from build123d import *

# Parameters (mm, degrees)
SKETCH015_W  = 9.5
SKETCH015_H  = 4.5
PAD007_DEPTH = 10
SKETCH014_W  = 0.5
SKETCH014_H  = 0.5
PAD008_DEPTH = 0.4
SKETCH017_W  = 0.5
SKETCH017_H  = 4.9
PAD010_DEPTH = 0.5


with BuildPart() as part:
    # Sketch015 → Pad007 (new body)
    with BuildSketch(Plane.XY):
        Rectangle(SKETCH015_W, SKETCH015_H)
    extrude(amount=PAD007_DEPTH)

    # Sketch014 (on Face3 of Pad007) → Pad008 (join)
    with BuildSketch(Plane.XZ.offset(2.25)):
        with Locations((-4.5, 9.75)):
            Rectangle(SKETCH014_W, SKETCH014_H)
        with Locations((4.5, 9.75)):
            Rectangle(SKETCH014_W, SKETCH014_H)
    extrude(amount=PAD008_DEPTH)

    # Sketch017 (on Face4 of Pad008) → Pad010 (join)
    with BuildSketch(Plane(origin=(0, 0, 0), x_dir=(1, 0, 0), z_dir=(0, 0, -1))):
        with Locations((-4.5, 0.2)):
            Rectangle(SKETCH017_W, SKETCH017_H)
        with Locations((4.5, 0.2)):
            Rectangle(SKETCH017_W, SKETCH017_H)
    extrude(amount=PAD010_DEPTH)


solid = part.part
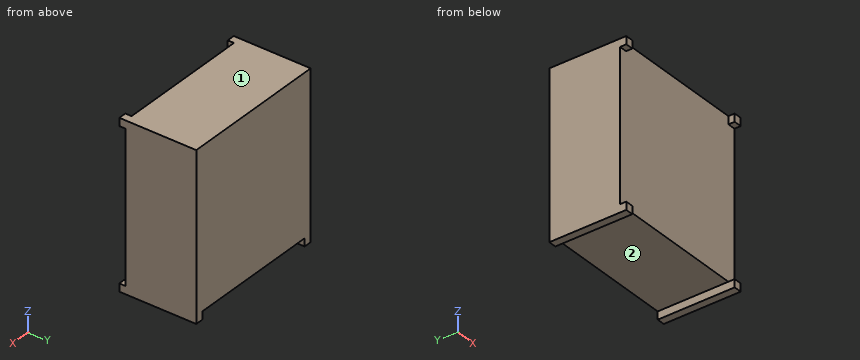
Could you check a few things on this model? Use its own coordinates, in mm. Face numbers are marked on the shaded views. A direction names the side the tool comes from. Round coordinates to 2 decimals unless told otherwise and drop trailing zeros. Loops run counter-clockwise (first coordinate to the right, second up) from the corner with the lowest first, then second, coordinate; pieces in that order, holes last. Notation, with made-up numbers: (54, 30.25) - (105, 30.25) arc R19 ccw to (105, 35.25) - close; hole circle Ø3 at (-17, 5.5). An arc over 180 degrees is marked (long way). Write item = value, one per line.
1) I need wall thicknesses on line 1 along Z through (x, y) = (-3.25, 2.05); line 2 along Y through (x, z) = (-0.25, 6.5). Which ranges of each line are inside material? Lowest first, please. Write a range as from..to.
Computed:
line_1 = 0..10
line_2 = -2.25..2.25
2) On a 3-axis mill with a long thin cutter (end or side, diameter ignored), from which of +Z, -Z, +X, -X, +Y, -Y can I reach the whole of each face in a straight line? I mean the marked faces 1 and 2. Say none if no direction works.
Computed:
face_1 = +Z, +X, -X, +Y, -Y
face_2 = -Z, +Y, -Y
3) Imagine slicing it at C-C (z = 5.25). Please give me the cut outline in (x, y), and give its area (4 significant figures).
Computed:
outline = (-4.75, -2.25) - (4.75, -2.25) - (4.75, 2.25) - (-4.75, 2.25) - close
area = 42.75 mm2
4) Imagine slicing it at A-A (y = -1.1). Please give me the cut outline in (x, z).
Computed:
outline = (-4.75, -0.5) - (-4.25, -0.5) - (-4.25, 0) - (4.25, 0) - (4.25, -0.5) - (4.75, -0.5) - (4.75, 10) - (-4.75, 10) - close
5) I'm going to push flat-ended pins straight in: P1, Ø2, axis at x = -0.5, y = 0, coming from the -Z side; P2, Ø1, axis at x = 3, z = 8, coming from the -Y side. Where does each tip first touch, or does it pass through?
Computed:
P1 = 0
P2 = -2.25
6) Imagine slicing it at B-B (x = 2). Please give me the cut outline in (y, z).
Computed:
outline = (-2.25, 0) - (2.25, 0) - (2.25, 10) - (-2.25, 10) - close
